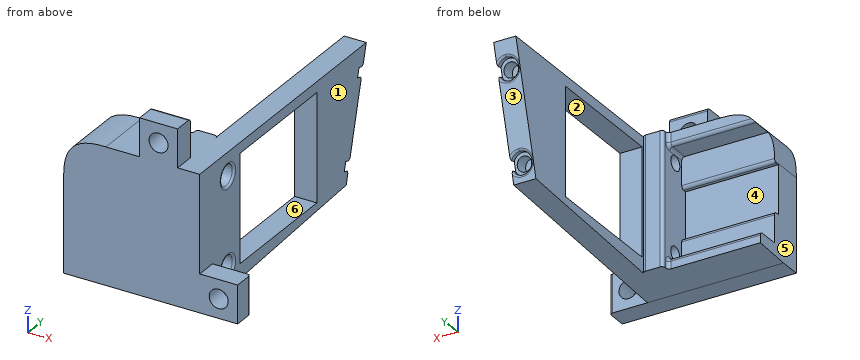
```python
from build123d import *

# Parameters (mm, degrees)
BOSS_EXTRUDE1_DEPTH = 11
SKETCH3_W           = 22
SKETCH3_H           = 3
BOSS_EXTRUDE2_DEPTH = 14
BOSS_EXTRUDE3_DEPTH = 5
SKETCH5_R           = 1.75
CUT_EXTRUDE1_DEPTH  = 36.096650541
SKETCH6_W           = 9
SKETCH6_H           = 9
BOSS_EXTRUDE4_DEPTH = 5
SKETCH10_R          = 2.25
CUT_EXTRUDE2_DEPTH  = 34.584744739
FILLET1_R           = 0.75
FILLET2_SIZE        = 10
SKETCH12_W          = 9
SKETCH12_H          = 32.0178
BOSS_EXTRUDE5_DEPTH = 65
CUT_EXTRUDE4_DEPTH  = 9
SKETCH14_R          = 2.5
CUT_EXTRUDE5_DEPTH  = 9.75
SKETCH15_R          = 1.7
CUT_EXTRUDE6_DEPTH  = 5
SKETCH16_R          = 2.5
CUT_EXTRUDE7_DEPTH  = 1.6
FILLET3_R           = 0.5
FILLET4_R           = 0.5
SKETCH17_W          = 3.75
SKETCH17_H          = 32.0178
CUT_EXTRUDE9_DEPTH  = 74.996250596
SKETCH18_W          = 9
SKETCH18_H          = 9
BOSS_EXTRUDE6_DEPTH = 5
CUT_EXTRUDE10_REACH = 73.697
SKETCH19_R          = 2.25
FILLET6_START       = -17
FILLET6_DEPTH       = 11
CUT_EXTRUDE11_REACH = 76.696
SKETCH20_W          = 25.5
SKETCH20_H          = 30
CUT_EXTRUDE12_DEPTH = 77.749642368


with BuildPart() as part:
    # Sketch1 → Boss-Extrude1 (new, symmetric)
    with BuildSketch(Plane(origin=(0, 0, 0), x_dir=(0, 0, -1), z_dir=(1, 0, 0))):
        Polygon((-13.0089, 0), (13.0089, 0), (13.0089, 8.5), (5.7589, 8.5), (5.7589, 7), (-5.7589, 7), (-5.7589, 8.5), (-13.0089, 8.5), align=None)
    extrude(amount=BOSS_EXTRUDE1_DEPTH, both=True)

    # Sketch3 → Boss-Extrude2 (add)
    with BuildSketch(Plane.XZ):
        with Locations((0, -14.5089)):
            Rectangle(SKETCH3_W, SKETCH3_H)
        with Locations((0, 14.5089)):
            Rectangle(SKETCH3_W, SKETCH3_H)
    extrude(amount=-BOSS_EXTRUDE2_DEPTH)

    # Sketch4 → Boss-Extrude3 (add)
    with BuildSketch(Plane(origin=(11, 0, 0), x_dir=(0, 0, -1), z_dir=(1, 0, 0))):
        Polygon((-8.8, 15.7), (-16.0089, 15.7), (-16.0089, 0), (16.0089, 0), (16.0089, 15.7), align=None)
    extrude(amount=BOSS_EXTRUDE3_DEPTH)

    # Sketch5 → Cut-Extrude1 (cut, through all)
    with BuildSketch(Plane(origin=(16, 0, 0), x_dir=(0, 0, -1), z_dir=(1, 0, 0))):
        with Locations((-10.5, 11)):
            Circle(SKETCH5_R)
        with Locations((10.5, 11)):
            Circle(SKETCH5_R)
    extrude(amount=-CUT_EXTRUDE1_DEPTH, mode=Mode.SUBTRACT)

    # Sketch6 → Boss-Extrude4 (add)
    with BuildSketch(Plane.XZ):
        with Locations((11.5, 20.5089)):
            Rectangle(SKETCH6_W, SKETCH6_H)
    extrude(amount=-BOSS_EXTRUDE4_DEPTH)

    # Sketch10 → Cut-Extrude2 (cut, through all)
    with BuildSketch(Plane.XZ):
        with Locations(Location((11.5, 20.5089, 0), (0, 0, 270))):
            Circle(SKETCH10_R)
    extrude(amount=-CUT_EXTRUDE2_DEPTH, mode=Mode.SUBTRACT)

    # Fillet1
    fillet1_edges = [part.edges().sort_by_distance(p)[0] for p in [
        (0, 8.5, 5.7589),
        (0, 8.5, -5.7589),
        (0, 14, -13.0089),
        (11, 14, -14.5089),
        (11, 11.25, -13.0089),
        (11, 14, 14.5089),
        (11, 11.25, 13.0089),
        (0, 14, 13.0089),
        (11, 15.7, 0),
        (16, 15.7, 0),
        (11.5, 5, 25.0089),
    ]]
    fillet(fillet1_edges, radius=FILLET1_R)

    # Fillet2
    # a fillet whose section is not a circle: 10 mm, written as the material it takes off along each edge
    with BuildSketch(Plane(origin=(-11, -25, 16.0089), x_dir=(0, 0, -1), z_dir=(0, 1, 0))) as fillet2_piece_1:
        with BuildLine():
            add(Edge.make_bspline([(FILLET2_SIZE, 0), (FILLET2_SIZE * 0.831801948466, 0), (FILLET2_SIZE * 0.663603896932, 0), (FILLET2_SIZE * 0.292893218813, -FILLET2_SIZE * 0.0716919198361), (FILLET2_SIZE * 0.0716919198361, -FILLET2_SIZE * 0.292893218813), (0, -FILLET2_SIZE * 0.663603896932), (0, -FILLET2_SIZE * 0.831801948466), (0, -FILLET2_SIZE)], knots=[0, 0, 0, 0, 0, 0, 0.5, 0.5, 1, 1, 1, 1, 1, 1], degree=5))
            Line((0, -FILLET2_SIZE), (0, 0))
            Line((0, 0), (FILLET2_SIZE, 0))
        make_face()
    extrude(amount=64, mode=Mode.SUBTRACT)

    # Sketch12 → Boss-Extrude5 (add)
    with BuildSketch(Plane.XZ):
        with Locations((20.5, 0)):
            Rectangle(SKETCH12_W, SKETCH12_H)
    extrude(amount=-BOSS_EXTRUDE5_DEPTH)

    # Sketch13 → Cut-Extrude4 (cut)
    with BuildSketch(Plane(origin=(25, 0, 0), x_dir=(0, 0, -1), z_dir=(1, 0, 0))):
        Polygon((16.0089, 65), (-16.0089, 65), (16.0089, 56.420856347), align=None)
    extrude(amount=-CUT_EXTRUDE4_DEPTH, mode=Mode.SUBTRACT)

    # Sketch14 → Cut-Extrude5 (cut)
    with BuildSketch(Plane(origin=(25, 0, 0), x_dir=(0, 0, -1), z_dir=(1, 0, 0))):
        with Locations((-10.5, 11)):
            Circle(SKETCH14_R)
        with Locations((10.5, 11)):
            Circle(SKETCH14_R)
    extrude(amount=-CUT_EXTRUDE5_DEPTH, mode=Mode.SUBTRACT)

    # Sketch15 → Cut-Extrude6 (cut)
    with BuildSketch(Plane(origin=(0, 56.643600623, -15.177607043), x_dir=(1, 0, 0), z_dir=(0, 0.9659258262890701, -0.25881904510251424))):
        with Locations(Location((19, -6.139382203, 0), (0, 0, 270))):
            Circle(SKETCH15_R)
        with Locations(Location((19, -26.139382203, 0), (0, 0, 270))):
            Circle(SKETCH15_R)
    extrude(amount=-CUT_EXTRUDE6_DEPTH, mode=Mode.SUBTRACT)

    # Sketch16 → Cut-Extrude7 (cut)
    with BuildSketch(Plane(origin=(0, 56.643600623, -15.177607043), x_dir=(1, 0, 0), z_dir=(0, 0.9659258262890701, -0.25881904510251424))):
        with Locations(Location((19, -6.139382203, 0), (0, 0, 270))):
            Circle(SKETCH16_R)
        with Locations(Location((19, -26.139382203, 0), (0, 0, 270))):
            Circle(SKETCH16_R)
    extrude(amount=-CUT_EXTRUDE7_DEPTH, mode=Mode.SUBTRACT)

    # Fillet3
    fillet3_edges = [part.edges().sort_by_distance(p)[0] for p in [
        (19, 57.58554205, -11.662233782),
        (19, 62.761922952, 7.656282744),
    ]]
    fillet(fillet3_edges, radius=FILLET3_R)

    # Fillet4
    fillet4_edges = [part.edges().sort_by_distance(p)[0] for p in [
        (25, 11, 13),
        (25, 11, -8),
    ]]
    fillet(fillet4_edges, radius=FILLET4_R)

    # Sketch17 → Cut-Extrude9 (cut, through all)
    with BuildSketch(Plane(origin=(0, 65, 0), x_dir=(-1, 0, 0), z_dir=(0, -1, 0))):
        with Locations((-23.125, 0)):
            Rectangle(SKETCH17_W, SKETCH17_H)
    extrude(amount=CUT_EXTRUDE9_DEPTH, mode=Mode.SUBTRACT)

    # Fillet5: read off the stored shape, not the designer's step
    # Fillet5 outline → Fillet5 (revolve, cut)
    with BuildSketch(Plane(origin=(0, 11, -10.5), x_dir=(0, 1, 0), z_dir=(0, 0, -1))):
        with BuildLine():
            ThreePointArc((2.5, 20.75), (2.646446609, 21.103553391), (3, 21.25))
            Line((3, 21.25), (2.5, 21.25))
            Line((2.5, 21.25), (2.5, 20.75))
        make_face()
    revolve(axis=Axis((0, 11, -10.5), (1, 0, 0)), mode=Mode.SUBTRACT)

    # Fillet5 2 outline → Fillet5 2 (revolve, cut)
    with BuildSketch(Plane(origin=(0, 11, 10.5), x_dir=(0, 1, 0), z_dir=(0, 0, -1))):
        with BuildLine():
            ThreePointArc((2.5, 20.75), (2.646446609, 21.103553391), (3, 21.25))
            Line((3, 21.25), (2.5, 21.25))
            Line((2.5, 21.25), (2.5, 20.75))
        make_face()
    revolve(axis=Axis((0, 11, 10.5), (1, 0, 0)), mode=Mode.SUBTRACT)

    # Sketch18 → Boss-Extrude6 (add)
    with BuildSketch(Plane.XZ):
        with Locations((25.75, -11.5089)):
            Rectangle(SKETCH18_W, SKETCH18_H)
    extrude(amount=-BOSS_EXTRUDE6_DEPTH)

    # Sketch19 → Cut-Extrude10 (cut, up to next)
    with BuildSketch(Plane(origin=(0, 5, 0), x_dir=(1, 0, 0), z_dir=(0, 1, 0)), mode=Mode.PRIVATE) as cut_extrude10_sk1:
        with Locations(Location((25.75, 11.5089, 0), (0, 0, 270))):
            Circle(SKETCH19_R)
    cut_extrude10_tool1 = extrude(cut_extrude10_sk1.sketch, amount=-CUT_EXTRUDE10_REACH, mode=Mode.PRIVATE) & part.part
    add(cut_extrude10_tool1.solids().sort_by_distance((25.75, 5, -11.5089))[0], mode=Mode.SUBTRACT)

    # Fillet6: read off the stored shape, not the designer's step
    # Fillet6 outline → Fillet6 (cut)
    with BuildSketch(Plane.XY.offset(FILLET6_START)):
        with BuildLine():
            ThreePointArc((29.5, 5), (30.030330086, 4.780330086), (30.25, 4.25))
            Line((30.25, 4.25), (30.25, 5))
            Line((30.25, 5), (29.5, 5))
        make_face()
    extrude(amount=FILLET6_DEPTH, mode=Mode.SUBTRACT)

    # Sketch20 → Cut-Extrude11 (cut, up to next)
    with BuildSketch(Plane.ZY.offset(-16), mode=Mode.PRIVATE) as cut_extrude11_sk1:
        with Locations((0.7411, 30.7)):
            Rectangle(SKETCH20_W, SKETCH20_H)
    cut_extrude11_tool1 = extrude(cut_extrude11_sk1.sketch, amount=-CUT_EXTRUDE11_REACH, mode=Mode.PRIVATE) & part.part
    add(cut_extrude11_tool1.solids().sort_by_distance((16, 30.7, 0.7411))[0], mode=Mode.SUBTRACT)

    # Sketch21 → Cut-Extrude12 (cut, through all)
    with BuildSketch(Plane(origin=(21.25, 0, 0), x_dir=(0, 0, -1), z_dir=(1, 0, 0))):
        Polygon((16.0089, 5), (16.0089, 56.420856347), (13.275665328, 57.15322437), align=None)
    extrude(amount=-CUT_EXTRUDE12_DEPTH, mode=Mode.SUBTRACT)


solid = part.part
```
Work out the finished part from the listing and answer in its coordinate system (mm). Face numbers are marked on the shaded views. A direction names the side the tool comes from. Give positions to 0.01 mm unless a question says otherwise; leave off trailing zeros. Order: outer loops, then holes, each group sorted by start corner. A loop starts at its lowest first (then second) coordinate and runs counter-clockwise, first axis right, second up. Notation, with made-up numbers: M 54,42 L 72,42 A18 ccw 72,77 Z; hole C 70.25,-6.5 d4. An arc over 180 degrees is marked long. Return JSON: item names as keys, results as strings.
1) Section C-C, the plane x = 2.5 is taken. Write down the section's boundary in (y, z).
Resolved:
{"outline": "M 0,-16.01 L 5,-16.01 L 14,-15.54 L 14,-13.76 A0.75 ccw 13.25,-13.01 L 8.5,-13.01 L 8.5,-6.51 A0.75 ccw 7.75,-5.76 L 7,-5.76 L 7,5.76 L 7.75,5.76 A0.75 ccw 8.5,6.51 L 8.5,13.01 L 13.25,13.01 A0.75 ccw 14,13.76 L 14,16.01 L 0,16.01 Z"}
2) Section D-D, the plane z = 10.5 is taken. Give the number of separate pieces and of enclosed holes in the cut face, plus the area to 3 significant figures.
Resolved:
{"separate pieces": "3", "enclosed holes": "0", "area": "373 mm^2"}
3) A tool of negligible diameter and unlimited length cuts with its end or side. For the marked faces 4, 5 and 6, from which of +Z, -Z, +X, -X, +Y, -Y can it reach the whole face along a straight path? Write none if from no direction.
Resolved:
{"face 4": "-X, +Y", "face 5": "+Z, -Z, -X, +Y, -Y", "face 6": "+X, -X"}
4) For a pull along Z with two mould halves and no side action, classify the marked faces 1, 2 and 3 as +Z half, -Z half, draft (parallel to the pull), parting line (faces both ways), or undercut.
Resolved:
{"face 1": "draft", "face 2": "undercut", "face 3": "-Z half"}
5) Section B-B, the plane z = 3.5 is taken. Write down the section's boundary in (x, y), plus the area to 3 significant figures.
Resolved:
{"outline": "M -11,0 L 21.25,0 L 21.25,15.7 L 16,15.7 L 16,14.95 A0.75 ccw 15.25,15.7 L 11.75,15.7 A0.75 ccw 11,14.95 L 11,7 L -11,7 Z; M 16,45.7 L 21.25,45.7 L 21.25,61.65 L 16,61.65 Z", "area": "398 mm^2"}
6) Each of these flat-tipped pins is pushed along its axis until it touches: pin 1 (2.5 mm diameter, centred on x = 18.5, y = 27.5, fed in from -Z); pin 2 (2 mm diameter, centred on x = -4, z = -15, fed in from +Y); pin 3 (12.5 mm diameter, centred on x = 4, z = 0, fed in from +Y). Where does it stop, or does it pass through?
Resolved:
{"pin 1": "z = -14.9", "pin 2": "y = 14", "pin 3": "y = 8.45"}
7) Straight lines are drawn through the part: line 1 along Y through (x, z) = (19.3, 10.5); line 2 along X through (y, z) = (16.5, -13); line 3 along X through (y, z) = (12, -4.5). For each, find the intervals that lie inside material, in ascending order. Write a range as [from, to].
Resolved:
{"line 1": "[0, 8.5], [13.5, 15.7], [45.7, 58.35]", "line 2": "[16, 21.25]", "line 3": "[11, 21.25]"}
8) Section A-A, the plane y = 39 is taken. Write down the section's boundary in (x, z), plus the area to 3 significant figures.
Resolved:
{"outline": "M 16,-14.23 L 21.25,-14.23 L 21.25,-12.01 L 16,-12.01 Z; M 16,13.49 L 21.25,13.49 L 21.25,16.01 L 16,16.01 Z", "area": "24.9 mm^2"}
